from build123d import *

# Parameters (mm, degrees)
EXTRUDE_1_DEPTH     = 38
SKETCH_2_R          = 2.5
CUT_EXTRUDE_1_DEPTH = 52.664784912
SKETCH_3_R          = 3
CUT_EXTRUDE_2_DEPTH = 53.490475326
CUT_EXTRUDE_3_DEPTH = 53.490475326


with BuildPart() as part:
    # 草图1 → 凸台-拉伸1 (new body)
    with BuildSketch(Plane.XY):
        with BuildLine():
            Line((0, 1), (0, 34.5))
            Line((0, 34.5), (-2, 34.5))
            Line((-2, 34.5), (-2, 3))
            ThreePointArc((-2, 3), (-2.292893219, 2.292893219), (-3, 2))
            Line((-3, 2), (-13, 2))
            Line((-13, 2), (-13, 0))
            Line((-13, 0), (-1, 0))
            ThreePointArc((-1, 0), (-0.292893219, 0.292893219), (0, 1))
        make_face()
    extrude(amount=EXTRUDE_1_DEPTH)

    # 草图2 → 切除-拉伸1 (cut, through all)
    with BuildSketch(Plane(origin=(0, 2, 0), x_dir=(1, 0, 0), z_dir=(0, 1, 0))):
        with Locations(Location((-7.5, -7.5, 0), (0, 0, 270))):
            Circle(SKETCH_2_R)
        with Locations(Location((-7.5, -30.5, 0), (0, 0, 90))):
            Circle(SKETCH_2_R)
    extrude(amount=-CUT_EXTRUDE_1_DEPTH, mode=Mode.SUBTRACT)

    # 草图3 → 切除-拉伸2 (cut, through all)
    with BuildSketch(Plane.ZY.offset(2)):
        with Locations((19, 27.5)):
            Circle(SKETCH_3_R)
    extrude(amount=-CUT_EXTRUDE_2_DEPTH, mode=Mode.SUBTRACT)

    # 草图4 → 切除-拉伸3 (cut, through all)
    with BuildSketch(Plane.ZY.offset(2)):
        with BuildLine():
            Line((0, 34.5), (0, 3.916925189))
            ThreePointArc((0, 3.916925189), (0.077442494, 4.594167854), (0.305771751, 5.23644561))
            Line((0.305771751, 5.23644561), (12.618411108, 30.376686151))
            ThreePointArc((12.618411108, 30.376686151), (15.201105625, 33.379489904), (19, 34.5))
            Line((19, 34.5), (0, 34.5))
        make_face()
        with BuildLine():
            Line((38, 34.5), (19, 34.5))
            ThreePointArc((19, 34.5), (22.798894375, 33.379489904), (25.381588892, 30.376686151))
            Line((25.381588892, 30.376686151), (37.694228249, 5.23644561))
            ThreePointArc((37.694228249, 5.23644561), (37.922557506, 4.594167854), (38, 3.916925189))
            Line((38, 3.916925189), (38, 34.5))
        make_face()
    extrude(amount=-CUT_EXTRUDE_3_DEPTH, mode=Mode.SUBTRACT)


solid = part.part
Model file for the job. Use its own axes, mm. A direction names the side the tool comes from. Give positions to 0.01 mm unless a question says otherwise; leave off trailing zeros. Loops run counter-clockwise (first coordinate to the right, second up) from the corner with the lowest first, then second, coordinate; pieces in that order, holes last.
1) Pull direction Z, two halves, no side cores. Call faces 3 (the flat face through (-7, 1, 0)), 4 (the cylindrical face through (-6, 1, 32.5)), 5 (the cylindrical face through (-0.301, 0.285, 18.734)): +Z half, -Z half, draft (parallel to the pull), parting line (faces both ways), or undercut.
2) Wall check: line 1 (X direction, y = 0.9, z = 7.5); line 2 (Y direction, x = -4.25, z = 6); line 3 (X direction, y = 11.5, z = 12). Give the ranges that are in metal, low to high.
3) Saw through at D-D (y = 27). Write the cut outline in (x, z), plus the area to 3 significant figures.
4) Saw through at B-B (z = 7.5). Write the cut outline in (x, y).
5) Saw through at C-C (x = -7.5). Write the cut outline in (y, z), plus the area to 3 significant figures.
6) Flat gauge pins, fed straight in: pin 1 Ø4 at (x, y) = (-5, 11.5) entering from -Z; pin 2 Ø12 at (y, z) = (8.5, 15) entering from +X; pin 3 Ø9.5 at (y, z) = (19, 23.5) entering from -X; pin 4 Ø4 at (x, z) = (-9, 21) entering from +Y. Where does each tip first touch, or does it go through?
7) Tool access for faces 1 (the cylindrical face through (-9.72, 1.01, 8.65)), 2 (the flat face through (-2, 15, 19)): list every direction of +Z, -Z, +X, -X, +Y, -Y with a clear straight run to the whole face (end or side of a thin tool).
8) Saw through at A-A (x = -1.5). Write the cut outline in (y, z), plus the area to 3 significant figures.
Answer block:
1. face 3: -Z half
1. face 4: undercut
1. face 5: draft
2. line 1: x = -13 to -10, -5 to -0.01
2. line 2: y = 0 to 2
2. line 3: x = -2 to 0
3. outline: (-2, 10.96) - (0, 10.96) - (0, 16.04) - (-2, 16.04) - close; (-2, 21.96) - (0, 21.96) - (0, 27.04) - (-2, 27.04) - close
3. area: 20.3 mm2
4. outline: (-13, 0) - (-10, 0) - (-10, 2) - (-13, 2) - close; (-5, 0) - (-1, 0) arc R1 ccw to (0, 1) - (0, 19.93) - (-2, 19.93) - (-2, 3) arc R1 cw to (-3, 2) - (-5, 2) - close
5. outline: (0, 0) - (2, 0) - (2, 5) - (0, 5) - close; (0, 10) - (2, 10) - (2, 28) - (0, 28) - close; (0, 33) - (2, 33) - (2, 38) - (0, 38) - close
5. area: 56.0 mm2
6. pin 1: passes through
6. pin 2: stops at x = 0
6. pin 3: stops at x = -2
6. pin 4: stops at y = 2
7. face 1: +Y, -Y
7. face 2: +Z, -Z, -X, +Y
8. outline: (0, 0) - (3.92, 0) arc R3 ccw to (5.24, 0.31) - (30.38, 12.62) arc R7 ccw to (30.38, 25.38) - (5.24, 37.69) arc R3 ccw to (3.92, 38) - (0, 38) - close; hole circle Ø6 at (27.5, 19)
8. area: 839 mm2
